```python
from build123d import *

# Parameters (mm, degrees)
CYLINDER001_R     = 4.1
CYLINDER001_DEPTH = 2
CYLINDER_R        = 6
CYLINDER_DEPTH    = 2


with BuildPart() as inner:
    # Cylinder001 → Cylinder001 (new body)
    with BuildSketch(Plane.XY):
        Circle(CYLINDER001_R)
    extrude(amount=CYLINDER001_DEPTH)


with BuildPart() as cut:
    # Cylinder → Cylinder (new body)
    with BuildSketch(Plane.XY):
        Circle(CYLINDER_R)
    extrude(amount=CYLINDER_DEPTH)

    # Cut: cut Inner
    add(inner.part, mode=Mode.SUBTRACT)


solid = cut.part
```
Geometry: final body of the model. Coordinates: model frame, mm. Coordinates: 2 decimals unless noted, no trailing zeros. Order: outer loops, then holes, each group sorted by start corner. A loop starts at its lowest first (then second) coordinate and runs counter-clockwise, first axis right, second up. Notation, with made-up numbers: M -27.5,5.25 L 16.5,5.25 A13 ccw 16.5,30.25 Z; hole C 48,72.5 d9. An arc over 180 degrees is marked long. Answer in a Markdown table with one row per item. Add a question column.
Q1. Section query C-C on z = 1.5. Return the cut outline in (x, y), and give its area (3 significant figures).
Q2. Line query: L1, parallel to Y at x = 0, z = 1.3; L2, parallel to Y at x = -3.5, z = 1; L3, parallel to X at y = -0.25, z = 0.6. Output: solid intervals per line, ascending.
Q3. Contact query for a flat-ended pin moving along its axis: P1, Ø2, axis at x = -2, y = -2.5, coming from the +Z side. Output: stop coordinate, or through.
Q4. Section query A-A on y = 0. Return the cut outline in (x, z).
Q5. Section query D-D on x = -4.25. Return the cut outline in (y, z), and give its area (3 significant figures).
Completed:
| question | item | result |
|---|---|---|
| 1 | outline | C 0,0 d12; hole C 0,0 d8.2 |
| 1 | area | 60.3 mm2 |
| 2 | L1 | y = -6 to -4.1, 4.1 to 6 |
| 2 | L2 | y = -4.87 to -2.14, 2.14 to 4.87 |
| 2 | L3 | x = -5.99 to -4.09, 4.09 to 5.99 |
| 3 | P1 | stops at z = 2 |
| 4 | outline | M -6,0 L -4.1,0 L -4.1,2 L -6,2 Z; M 4.1,0 L 6,0 L 6,2 L 4.1,2 Z |
| 5 | outline | M -4.24,0 L 4.24,0 L 4.24,2 L -4.24,2 Z |
| 5 | area | 16.9 mm2 |
